Read the model definition and answer for the solid it produces. Units are mm, in the model's axes. Give positions to 0.01 mm unless a question says otherwise; leave off trailing zeros. Write each loop counter-clockwise with the first axis right and the second up, starting at its lowest first coordinate (ties: lowest second). Pieces come first, ordered by that corner, then holes. Notation, with made-up numbers: M 42.5,45.5 L 55.5,45.5 A22 cw 55.5,81.5 Z; hole C -16,-35.75 d11. An arc over 180 degrees is marked long. Use a Markdown table: item, result. Add a question column.
Item 1: A cutting plane is placed at B-B on z = 165. Determine the outline of the cut face in (x, y).
Item 2: Given P1, Ø2.5, axis at x = 13, y = 0.5, coming from the +Z side; P2, Ø4, axis at y = -4, z = 181.5, coming from the +X side; P3, Ø8, axis at x = -11, z = 49.5, coming from the -Y side; P4, Ø10.5, axis at x = 0, y = 0, coming from the -Z side, each flat-ended and moving along its own axis, determine where each tip first touches the part or whether it passes through.
Item 3: A cutting plane is placed at A-A on x = 0. Determine the outline of the cut face in (y, z).
Item 4: Consider probe 1 along Y at (x, z) = (0, 43.5); probe 2 along X at (y, z) = (-3.75, 53.5). Determine where each line is inside the solid, lowest interval first. Write a range as [from, to].
from build123d import *

# Parameters (mm, degrees)
F0_R     = 8.65
F1_DEPTH = 203.2
F2_R     = 1.6
F3_DEPTH = 5


with BuildPart() as f1:
    # F0 (on Top) → F1 (new body)
    with BuildSketch(Plane.XY):
        with BuildLine():
            Line((11.736521, -2.426381), (11.736521, 2.500816))
            ThreePointArc((11.736521, 2.500816), (0, 12), (-11.736521, 2.500816))
            Line((-11.736521, 2.500816), (-11.736521, -2.426381))
            Line((-11.736521, -2.426381), (-11.752135, -2.426381))
            ThreePointArc((-11.752135, -2.426381), (0, -12), (11.752135, -2.426381))
            Line((11.752135, -2.426381), (11.736521, -2.426381))
        make_face()
        Circle(F0_R, mode=Mode.SUBTRACT)
        with BuildLine():
            Line((-11.736521, -2.426381), (-11.736521, 2.500816))
            ThreePointArc((-11.736521, 2.500816), (-11.99994, 0.038028), (-11.752135, -2.426381))
            Line((-11.752135, -2.426381), (-11.736521, -2.426381))
        make_face()
        with BuildLine():
            ThreePointArc((11.752135, -2.426381), (11.937873, -1.219504), (12, 0))
            ThreePointArc((12, 0), (11.933948, 1.257329), (11.736521, 2.500816))
            Line((11.736521, 2.500816), (11.736521, -2.426381))
            Line((11.736521, -2.426381), (11.752135, -2.426381))
        make_face()
    extrude(amount=F1_DEPTH)

    # F2
    f2_edges = [f1.edges().sort_by_distance(p)[0] for p in [
        (-11.752135, 2.426381, 203.2),
        (-8.65, 0, 203.2),
    ]]
    fillet(f2_edges, radius=F2_R)

    # F0 (on Top) → F3 (join)
    with BuildSketch(Plane.XY):
        with BuildLine():
            ThreePointArc((11.736521, 2.500816), (11.933948, 1.257329), (12, 0))
            ThreePointArc((12, 0), (11.937873, -1.219504), (11.752135, -2.426381))
            Line((11.752135, -2.426381), (13.798083, -2.426381))
            Line((13.798083, -2.426381), (13.798083, 2.500816))
            Line((13.798083, 2.500816), (11.736521, 2.500816))
        make_face()
        with BuildLine():
            ThreePointArc((-11.752135, -2.426381), (-11.99994, 0.038028), (-11.736521, 2.500816))
            Line((-11.736521, 2.500816), (-13.798083, 2.500816))
            Line((-13.798083, 2.500816), (-13.798083, -2.426381))
            Line((-13.798083, -2.426381), (-11.752135, -2.426381))
        make_face()
    extrude(amount=F3_DEPTH)


solid = f1.part
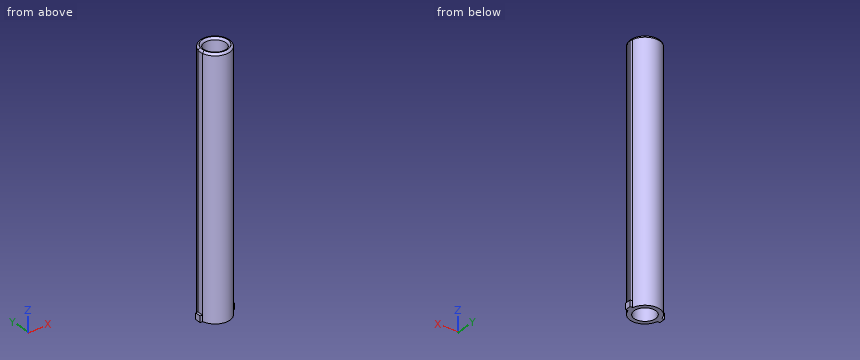
Filled in:
| question | item | result |
|---|---|---|
| 1 | outline | M -11.75,-2.43 A12 ccw 11.75,-2.43 A12 ccw 12,0 A12 ccw 11.74,2.5 A12 ccw -11.74,2.5 A12 ccw Z; hole C 0,0 d17.3 |
| 2 | P1 | z = 202.44 |
| 2 | P2 | x = 11.83 |
| 2 | P3 | y = -9.75 |
| 2 | P4 | through |
| 3 | outline | M -12,0 L -8.65,0 L -8.65,201.6 A1.6 ccw -10.25,203.2 L -10.4,203.2 A1.6 ccw -12,201.6 Z; M 8.65,0 L 12,0 L 12,201.6 A1.6 ccw 10.4,203.2 L 10.25,203.2 A1.6 ccw 8.65,201.6 Z |
| 4 | probe 1 | [-12, -8.65], [8.65, 12] |
| 4 | probe 2 | [-11.4, -7.79], [7.79, 11.4] |
